```python
from build123d import *

# Parameters (mm, degrees)
SKETCH2_W            = 15.8
SKETCH2_H            = 15.8
BOSS_EXTRUDE2_DEPTH  = 5.4
SKETCH4_W            = 13.4
SKETCH4_H            = 13.4
CUT_EXTRUDE1_DEPTH   = 3.2
SKETCH7_R            = 3.265
SKETCH7_R_2          = 2.4
BOSS_EXTRUDE5_DEPTH  = 3.2
SKETCH8_R            = 5.15
CUT_EXTRUDE2_DEPTH   = 0.3
BOSS_EXTRUDE8_DEPTH  = 2.8
BOSS_EXTRUDE11_DEPTH = 2.7
CIRPATTERN1_COUNT    = 4


with BuildPart() as part:
    # Sketch2 → Boss-Extrude2 (new body)
    with BuildSketch(Plane(origin=(0, 0, 0), x_dir=(1, 0, 0), z_dir=(0, 1, 0))):
        with Locations((7.9, 7.9)):
            Rectangle(SKETCH2_W, SKETCH2_H)
    extrude(amount=-BOSS_EXTRUDE2_DEPTH)

    # Sketch4 → Cut-Extrude1 (cut)
    with BuildSketch(Plane(origin=(0, 0, 0), x_dir=(1, 0, 0), z_dir=(0, 1, 0))):
        with Locations((7.9, 7.9)):
            Rectangle(SKETCH4_W, SKETCH4_H)
    extrude(amount=-CUT_EXTRUDE1_DEPTH, mode=Mode.SUBTRACT)

    # Sketch7 → Boss-Extrude5 (add)
    with BuildSketch(Plane(origin=(0, -3.2, 0), x_dir=(1, 0, 0), z_dir=(0, 1, 0))):
        with Locations((7.85, 7.85)):
            Circle(SKETCH7_R)
        with Locations((7.85, 7.85)):
            Circle(SKETCH7_R_2, mode=Mode.SUBTRACT)
    extrude(amount=BOSS_EXTRUDE5_DEPTH)

    # Sketch8 → Cut-Extrude2 (cut)
    with BuildSketch(Plane(origin=(0, -5.4, 0), x_dir=(-1, 0, 0), z_dir=(0, -1, 0))):
        with Locations((-7.9, 7.9)):
            Circle(SKETCH8_R)
    extrude(amount=-CUT_EXTRUDE2_DEPTH, mode=Mode.SUBTRACT)

    # Sketch11 → Boss-Extrude8 (add)
    with BuildSketch(Plane.XZ.offset(5.4)):
        Polygon((11.683021279, -2.207790411), (12.637615434, -3.162384566), (13.203300859, -2.596699141), (12.248706704, -1.642104986), align=None)
        with BuildLine():
            ThreePointArc((11.585853022, -2.304958669), (12.133497372, -2.706975833), (12.637615434, -3.162384566))
            Line((12.637615434, -3.162384566), (11.683021279, -2.207790411))
            Line((11.683021279, -2.207790411), (11.585853022, -2.304958669))
        make_face()
        with BuildLine():
            ThreePointArc((10.459662524, -3.431149167), (11.028098464, -3.808851017), (11.541599923, -4.258400077))
            Line((11.541599923, -4.258400077), (12.637615434, -3.162384566))
            ThreePointArc((12.637615434, -3.162384566), (12.133497372, -2.706975833), (11.585853022, -2.304958669))
            Line((11.585853022, -2.304958669), (10.459662524, -3.431149167))
        make_face()
        with BuildLine():
            Line((12.637615434, -3.162384566), (11.541599923, -4.258400077))
            ThreePointArc((11.541599923, -4.258400077), (11.991148983, -4.771901536), (12.368850833, -5.340337476))
            Line((12.368850833, -5.340337476), (13.495041331, -4.214146978))
            ThreePointArc((13.495041331, -4.214146978), (13.093024167, -3.666502628), (12.637615434, -3.162384566))
        make_face()
        with BuildLine():
            Line((13.592209589, -4.116978721), (12.637615434, -3.162384566))
            ThreePointArc((12.637615434, -3.162384566), (13.093024167, -3.666502628), (13.495041331, -4.214146978))
            Line((13.495041331, -4.214146978), (13.592209589, -4.116978721))
        make_face()
        Polygon((13.203300859, -2.596699141), (12.637615434, -3.162384566), (13.592209589, -4.116978721), (14.157895014, -3.551293296), align=None)
    boss_extrude8 = extrude(amount=BOSS_EXTRUDE8_DEPTH)

    # Sketch29 → Boss-Extrude11 (add)
    with BuildSketch(Plane(origin=(6.945405845, 0, -6.945405845), x_dir=(0.707106781, 0, 0.707106781), z_dir=(-0.707106781, 0, 0.707106781))):
        Polygon((7.5, -8.2), (7.5, -5.4), (8.4, -5.4), align=None)
    boss_extrude11 = extrude(amount=-BOSS_EXTRUDE11_DEPTH)

    # CirPattern1: Boss-Extrude8, Boss-Extrude11 ×4 about axis
    cirpattern1_axis = Axis((7.9, 0, -7.9), (0, 1, 0))
    for i in range(1, CIRPATTERN1_COUNT):
        add(boss_extrude8.rotate(cirpattern1_axis, i * 360 / CIRPATTERN1_COUNT))
        add(boss_extrude11.rotate(cirpattern1_axis, i * 360 / CIRPATTERN1_COUNT))


solid = part.part
```
Part model, mm, in its own coordinate system. A direction names the side the tool comes from. Coordinates: 2 decimals unless noted, no trailing zeros. Loops run counter-clockwise (first coordinate to the right, second up) from the corner with the lowest first, then second, coordinate; pieces in that order, holes last. Notation, with made-up numbers: (21.5, 67) - (58.5, 67) arc R14 cw to (58.5, 74) - close; hole circle Ø5 at (79, 16.5). An arc over 180 degrees is marked (long way). Write item = value, one per line. Start each with the question number.
Item 1: Cut at A-A, the plane y = -1.5. Give the cut face in (x, z) (3 decimals).
Item 2: Mould opens along Z. For faces 1 (the flat face through (8, -3, 0)), 2 (the cylindrical face through (7.33, -1.622, -5.507)), 3 (the flat face through (0, -3, -8)), 4 (the flat face through (2.29, -6.78, -13.54)) say: released by +Z, released by -Z, zero draft, split by the parting line, or undercut.
Item 3: Cut at C-C, the plane x = 7.9. Give the cut face in (y, z).
Item 4: Wall check: L1, parallel to Z at x = 7.85, y = -1.4 (3 decimals); L2, parallel to X at y = -5.2, z = -7.9; L3, parallel to Z at x = 14, y = -0.25. Give the ranges that are in metal, low to high. Write a range as from..to.
Item 5: Cut at B-B, the plane z = -6. Give the cut face in (x, y).
Item 6: Flat gauge pin, fed straight in: pin 1 Ø3 at (x, z) = (7.85, -7.85) entering from -Y. Where does the tip first touch, or does it go through?
Item 7: Cut at D-D, the plane y = -6.5. Give the cut face in (x, z).
Item 8: 3-axis set-ups, long thin cutter, end or side, ignore diameter. For faces 5 (the flat face through (8, -2, -1.2)), 6 (the flat face through (7.8, -5.4, -13.3)), 7 (the flat face through (1, 0, -8)): which of +Z, -Z, +X, -X, +Y, -Y reach the whole face in a straight line?
The answers:
q1.outline = (0, -15.8) - (15.8, -15.8) - (15.8, 0) - (0, 0) - close; circle Ø6.53 at (7.85, -7.85); hole (1.2, -14.6) - (14.6, -14.6) - (14.6, -1.2) - (1.2, -1.2) - close; hole circle Ø4.8 at (7.85, -7.85)
q2.face_1 = released by +Z
q2.face_2 = undercut
q2.face_3 = zero draft
q2.face_4 = released by -Z
q3.outline = (-5.4, -15.8) - (0, -15.8) - (0, -14.6) - (-3.2, -14.6) - (-3.2, -11.11) - (0, -11.11) - (0, -10.25) - (-3.2, -10.25) - (-3.2, -5.45) - (0, -5.45) - (0, -4.59) - (-3.2, -4.59) - (-3.2, -1.2) - (0, -1.2) - (0, 0) - (-5.4, 0) - (-5.4, -2.75) - (-5.1, -2.75) - (-5.1, -13.05) - (-5.4, -13.05) - close
q4.L1 = -15.8..-14.6, -11.115..-10.25, -5.45..-4.585, -1.2..0
q4.L2 = 0..2.75, 13.05..15.8
q4.L3 = -15.8..-14.6, -1.2..0
q5.outline = (0, -5.4) - (3.11, -5.4) - (3.11, -5.1) - (12.69, -5.1) - (12.69, -5.4) - (15.8, -5.4) - (15.8, 0) - (14.6, 0) - (14.6, -3.2) - (10.54, -3.2) - (10.54, 0) - (9.38, 0) - (9.38, -3.2) - (6.32, -3.2) - (6.32, 0) - (5.16, 0) - (5.16, -3.2) - (1.2, -3.2) - (1.2, 0) - (0, 0) - close
q6.pin_1 = -5.1
q7.outline = (1.26, -12.64) - (3.16, -14.54) - (5.34, -12.37) arc R5.15 cw to (3.43, -10.46) - close; (1.26, -3.16) - (3.43, -5.34) arc R5.15 cw to (5.34, -3.43) - (3.16, -1.26) - close; (10.46, -12.37) - (12.64, -14.54) - (14.54, -12.64) - (12.37, -10.46) arc R5.15 cw to start; (10.46, -3.43) arc R5.15 cw to (12.37, -5.34) - (14.54, -3.16) - (12.64, -1.26) - close
q8.face_5 = +Y
q8.face_6 = -Y
q8.face_7 = +Z, -Z, +X, -X, +Y
